Design review of the part shown in the three views and the two pictorial views. Dimensions are in mm from the part's minimum x, y and z. Coordinates: 2 decimals unless noted, no trailing zeros. Loops run counter-clockwise (first coordinate to the right, second up) from the corner with the lowest first, then second, coordinate; pieces in that order, holes last. Notation, with made-up numbers: (6, 18.5) -> (36, 18.5) arc R32 ccw to (36, 55.5) -> close; hole circle Ø1 at (29, 69). An arc over 180 degrees is marked (long way). Use a Markdown table: item, result. Add a question column.
Q1. Take a section at B-B on z = 12.7. Write out the cut boundary in (x, y), plus the area to 3 significant figures.
Q2. For probe 1 along Y at (x, z) = (8.5, 12.7); probe 2 along Z at (x, y) = (4.5, 63.5) (1 decimal); probe 3 along Z at (x, y) = (1.75, 12) (1 decimal), list the stretches that pass through material, from the lowest coordinate up.
Q3. Take a section at A-A on y = 12.7. Write out the cut boundary in (x, z) (1 decimal), plus the area to 3 significant figures.
Q4. Clearance check with a flat-ended pin moving along its axis: pin 1 Ø4 at (y, z) = (63.5, 12.7) entering from +X. State where the tip first meets the part, or that it passes through.
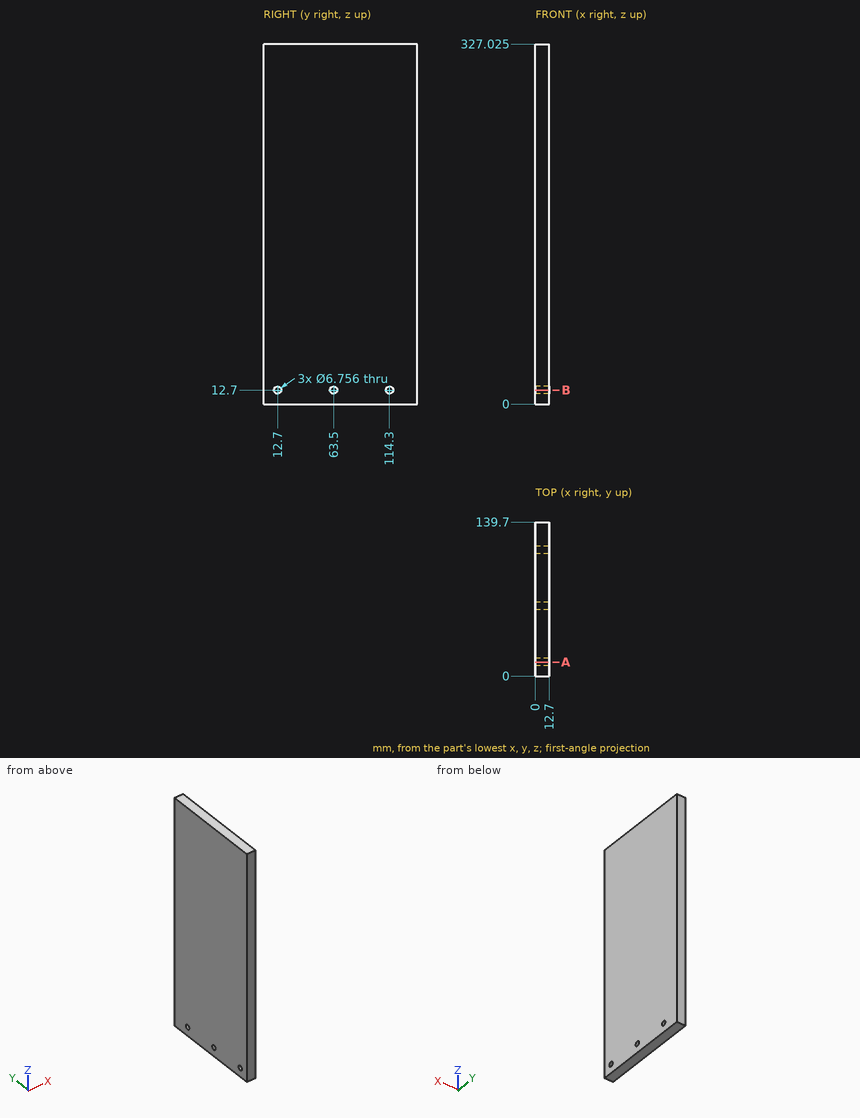
Answer list:
| question | item | result |
|---|---|---|
| 1 | outline | (0, 0) -> (12.7, 0) -> (12.7, 9.32) -> (0, 9.32) -> close; (0, 16.08) -> (12.7, 16.08) -> (12.7, 60.12) -> (0, 60.12) -> close; (0, 66.88) -> (12.7, 66.88) -> (12.7, 110.92) -> (0, 110.92) -> close; (0, 117.68) -> (12.7, 117.68) -> (12.7, 139.7) -> (0, 139.7) -> close |
| 1 | area | 1,520 mm² |
| 2 | probe 1 | 0 to 9.32, 16.08 to 60.12, 66.88 to 110.92, 117.68 to 139.7 |
| 2 | probe 2 | 0 to 9.3, 16.1 to 327 |
| 2 | probe 3 | 0 to 9.4, 16 to 327 |
| 3 | outline | (0, 0) -> (12.7, 0) -> (12.7, 9.3) -> (0, 9.3) -> close; (0, 16.1) -> (12.7, 16.1) -> (12.7, 327) -> (0, 327) -> close |
| 3 | area | 4,070 mm² |
| 4 | pin 1 | through |
